Design review of the part built by this model. Coordinates are the model's own, in mm. Face numbers are marked on the shaded views. Coordinates: 2 decimals unless noted, no trailing zeros. Write each loop counter-clockwise with the first axis right and the second up, starting at its lowest first coordinate (ties: lowest second). Pieces come first, ordered by that corner, then holes. Notation, with made-up numbers: (56, -28.5) -> (103, -28.5) arc R19 cw to (103, -6.5) -> close; hole circle Ø10 at (-31.5, -13.75). An arc over 180 degrees is marked (long way). One line per question, with ' | ' between items. Start each with the question number.
Q1. For P1, Ø5, axis at x = 0, y = 5, coming from the +Z side; P2, Ø1.9, axis at x = 0, y = 5, coming from the -Z side; P3, Ø12, axis at y = 5.5, z = -12, coming from the +X side, all flat-tipped, find the tip position at first contact; note any pin that passes through.
Q2. Add section A-A on x = 0. Give the number of separate pieces and of enclosed holes in the cut face, and give its area (3 significant figures).
Q3. Wall thickness on probe 1 along Y at (x, z) = (0, -3.3) (3 decimals); probe 2 along Y at (x, z) = (0, -10.5) (3 decimals); probe 3 along X at (y, z) = (2.75, 0): over which ranges is each line inside the solid? List them lowest first.
Q4. Add section D-D on y = 12.25. State the section outline as (x, z) points, and give its area (3 significant figures).
Q5. Add section C-C on x = 7.5. State the section outline as (y, z) points.
Q6. Draft analysis for pull direction X (two halves, no side actions). For the marked faces 1, 2 and 3, state which applies: pulls with the +X half, pulls with the -X half, needs draft (parallel to the pull), parting line crosses it, or undercut.
Q7. Add section B-B on z = 0. State the section outline as (x, y) points.
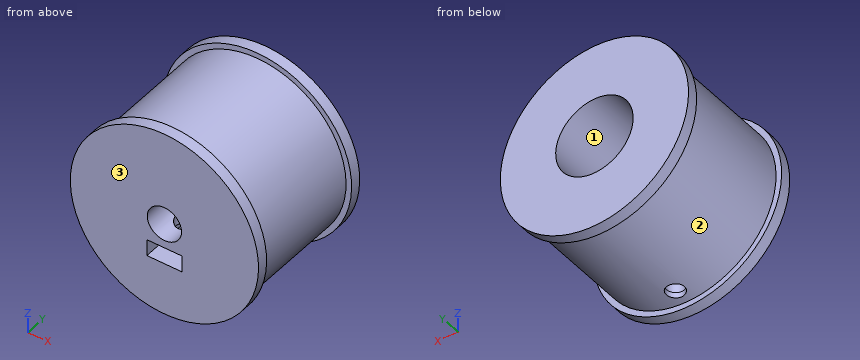
from build123d import *

# Parameters (mm, degrees)
CROQUIS1_R                 = 15
CROQUIS1_R_2               = 3
SALIENTE_EXTRUIR1_DEPTH    = 25
CROQUIS2_R                 = 16.5
CROQUIS2_R_2               = 3
SALIENTE_EXTRUIR2_DEPTH    = 2
SALIENTE_EXTRUIR3_START    = -2
CROQUIS3_R                 = 16.5
CROQUIS3_R_2               = 3
SALIENTE_EXTRUIR3_DEPTH    = 2
CORTAR_EXTRUIR1_REACH      = 36.198
CORTAR_EXTRUIR1_END_RADIUS = 15
CROQUIS4_R                 = 1.625
CROQUIS5_R                 = 7
CORTAR_EXTRUIR2_DEPTH      = 16
CORTAR_EXTRUIR3_DEPTH      = 9
SALIENTE_EXTRUIR5_START    = 21
CROQUIS10_R                = 16
CROQUIS10_R_2              = 15
SALIENTE_EXTRUIR5_DEPTH    = 21
SALIENTE_EXTRUIR6_START    = -2
CROQUIS12_R                = 17
CROQUIS12_R_2              = 16
SALIENTE_EXTRUIR6_DEPTH    = 2
CROQUIS13_R                = 17
CROQUIS13_R_2              = 16
SALIENTE_EXTRUIR7_DEPTH    = 2
CROQUIS14_R                = 3.1
CORTAR_EXTRUIR4_DEPTH      = 10
CROQUIS15_R                = 1.625
CORTAR_EXTRUIR5_DEPTH      = 9


with BuildPart() as part:
    # Croquis1 → Saliente-Extruir1 (new body)
    with BuildSketch(Plane(origin=(0, 0, 0), x_dir=(1, 0, 0), z_dir=(0, 1, 0))):
        with Locations(Location((0, 0, 0), (0, 0, 270))):
            Circle(CROQUIS1_R)
        with Locations(Location((0, 0, 0), (0, 0, 270))):
            Circle(CROQUIS1_R_2, mode=Mode.SUBTRACT)
    extrude(amount=SALIENTE_EXTRUIR1_DEPTH)

    # Croquis2 → Saliente-Extruir2 (add)
    with BuildSketch(Plane.XZ):
        with Locations(Location((0, 0, 0), (0, 0, 270))):
            Circle(CROQUIS2_R)
        with Locations(Location((0, 0, 0), (0, 0, 90))):
            Circle(CROQUIS2_R_2, mode=Mode.SUBTRACT)
    extrude(amount=-SALIENTE_EXTRUIR2_DEPTH)

    # Croquis3 → Saliente-Extruir3 (add)
    with BuildSketch(Plane(origin=(0, 25, 0), x_dir=(1, 0, 0), z_dir=(0, 1, 0)).offset(SALIENTE_EXTRUIR3_START)):
        with Locations(Location((0, 0, 0), (0, 0, 90))):
            Circle(CROQUIS3_R)
        with Locations(Location((0, 0, 0), (0, 0, 270))):
            Circle(CROQUIS3_R_2, mode=Mode.SUBTRACT)
    extrude(amount=SALIENTE_EXTRUIR3_DEPTH)

    # Cortar-Extruir1: up to this cylinder (the profile starts inside it)
    cortar_extruir1_end = Plane(origin=(0, 5, 0), z_dir=(0, -1, 0)) * Cylinder(CORTAR_EXTRUIR1_END_RADIUS, 103.396, mode=Mode.PRIVATE)
    # Croquis4 → Cortar-Extruir1 (cut, up to the surface)
    with BuildSketch(Plane.XY, mode=Mode.PRIVATE) as cortar_extruir1_sk1:
        with Locations((0, 5)):
            Circle(CROQUIS4_R)
    cortar_extruir1_tool1 = extrude(cortar_extruir1_sk1.sketch, amount=-CORTAR_EXTRUIR1_REACH, mode=Mode.PRIVATE) & cortar_extruir1_end
    add(cortar_extruir1_tool1.solids().sort_by_distance((0, 5, 0))[0], mode=Mode.SUBTRACT)

    # Croquis5 → Cortar-Extruir2 (cut)
    with BuildSketch(Plane(origin=(0, 25, 0), x_dir=(1, 0, 0), z_dir=(0, 1, 0))):
        with Locations(Location((0, 0, 0), (0, 0, 270))):
            Circle(CROQUIS5_R)
    extrude(amount=-CORTAR_EXTRUIR2_DEPTH, mode=Mode.SUBTRACT)

    # Croquis7 → Cortar-Extruir3 (cut)
    with BuildSketch(Plane.XZ):
        Polygon((-3.17, -7.5), (3.17, -7.5), (3.17, -4.5), (0, -4.5), (-3.17, -4.5), align=None)
    extrude(amount=-CORTAR_EXTRUIR3_DEPTH, mode=Mode.SUBTRACT)

    # Croquis10 → Saliente-Extruir5 (add)
    with BuildSketch(Plane.XZ.offset(-23).offset(SALIENTE_EXTRUIR5_START)):
        with Locations(Location((0, 0, 0), (0, 0, 90))):
            Circle(CROQUIS10_R)
        Circle(CROQUIS10_R_2, mode=Mode.SUBTRACT)
    extrude(amount=-SALIENTE_EXTRUIR5_DEPTH)

    # Croquis12 → Saliente-Extruir6 (add)
    with BuildSketch(Plane(origin=(0, 2, 0), x_dir=(1, 0, 0), z_dir=(0, 1, 0)).offset(SALIENTE_EXTRUIR6_START)):
        with Locations(Location((0, 0, 0), (0, 0, 270))):
            Circle(CROQUIS12_R)
        with Locations(Location((0, 0, 0), (0, 0, 270))):
            Circle(CROQUIS12_R_2, mode=Mode.SUBTRACT)
    extrude(amount=SALIENTE_EXTRUIR6_DEPTH)

    # Croquis13 → Saliente-Extruir7 (add)
    with BuildSketch(Plane.XZ.offset(-23)):
        with Locations(Location((0, 0, 0), (0, 0, 90))):
            Circle(CROQUIS13_R)
        with Locations(Location((0, 0, 0), (0, 0, 90))):
            Circle(CROQUIS13_R_2, mode=Mode.SUBTRACT)
    extrude(amount=-SALIENTE_EXTRUIR7_DEPTH)

    # Croquis14 → Cortar-Extruir4 (cut)
    with BuildSketch(Plane.XZ):
        with Locations(Location((0, 0, 0), (0, 0, 270))):
            Circle(CROQUIS14_R)
    extrude(amount=-CORTAR_EXTRUIR4_DEPTH, mode=Mode.SUBTRACT)

    # Croquis15 → Cortar-Extruir5 (cut)
    with BuildSketch(Plane.XY.offset(-7.5)):
        with Locations((0, 5)):
            Circle(CROQUIS15_R)
    extrude(amount=-CORTAR_EXTRUIR5_DEPTH, mode=Mode.SUBTRACT)


solid = part.part
Output values:
1) P1: stops at z = 16 | P2: stops at z = 2.95 | P3: stops at x = 15.43
2) separate pieces: 5 | enclosed holes: 0 | area: 469 mm2
3) probe 1: y = 0 to 3.375, 6.625 to 9 | probe 2: y = 0 to 3.375, 6.625 to 25 | probe 3: x = -16 to -3.1, 3.1 to 16
4) outline: circle Ø32 at (0, 0); hole circle Ø14 at (0, 0) | area: 650 mm2
5) outline: (0, -15.26) -> (2, -15.26) -> (2, -14.13) -> (23, -14.13) -> (23, -15.26) -> (25, -15.26) -> (25, 15.26) -> (23, 15.26) -> (23, 14.13) -> (2, 14.13) -> (2, 15.26) -> (0, 15.26) -> close
6) face 1: undercut | face 2: parting line crosses it | face 3: needs draft
7) outline: (-17, 0) -> (-3.1, 0) -> (-3.1, 9) -> (-7, 9) -> (-7, 25) -> (-17, 25) -> (-17, 23) -> (-16, 23) -> (-16, 2) -> (-17, 2) -> close; (3.1, 0) -> (17, 0) -> (17, 2) -> (16, 2) -> (16, 23) -> (17, 23) -> (17, 25) -> (7, 25) -> (7, 9) -> (3.1, 9) -> close
